```python
from build123d import *

# Parameters (mm, degrees)
SKETCH1_R           = 1
BOSS_EXTRUDE1_DEPTH = 12
SKETCH2_R           = 3.3
CUT_EXTRUDE1_DEPTH  = 4.5
FILLET1_R           = 1
FILLET2_R           = 1
FILLET3_R           = 1
FILLET6_R           = 1


with BuildPart() as part:
    # Sketch1 → Boss-Extrude1 (new body)
    with BuildSketch(Plane.XY):
        with BuildLine():
            Line((0.332668694, 15.169303239), (0.332668694, 22.304947181))
            ThreePointArc((0.332668694, 22.304947181), (-0.167437886, 27.468747249), (4.56623438, 25.3457106))
            Line((4.56623438, 25.3457106), (41.53945423, 8.884172534))
            ThreePointArc((41.53945423, 8.884172534), (44.223987307, 10.459606893), (47.320366603, 10.141571494))
            ThreePointArc((47.320366603, 10.141571494), (47.827175417, 8.821289393), (46.506893317, 8.314480578))
            ThreePointArc((46.506893317, 8.314480578), (42.546047014, 6.794054135), (44.066473458, 2.833207832))
            ThreePointArc((44.066473458, 2.833207832), (44.573282273, 1.512925732), (43.253000172, 1.006116917))
            ThreePointArc((43.253000172, 1.006116917), (40.944771655, 3.094367949), (40.319244301, 6.143536161))
            Line((40.319244301, 6.143536161), (5.332668694, 21.720563222))
            Line((5.332668694, 21.720563222), (5.332668694, 12.544828977))
            Line((5.332668694, 12.544828977), (17.953063304, 7.445858574))
            Line((17.953063304, 7.445858574), (16.829243524, 4.66430701))
            Line((16.829243524, 4.66430701), (3.42965312, 10.078092949))
            ThreePointArc((3.42965312, 10.078092949), (-0.980376986, 10.883023916), (0.332668694, 15.169303239))
        make_face()
        with Locations((1.582668694, 25.03212521)):
            Circle(SKETCH1_R, mode=Mode.SUBTRACT)
        with Locations((1.582668694, 12.44212521)):
            Circle(SKETCH1_R, mode=Mode.SUBTRACT)
    extrude(amount=BOSS_EXTRUDE1_DEPTH)

    # Sketch2 → Cut-Extrude1 (cut)
    with BuildSketch(Plane.XY.offset(12)):
        with Locations((1.582668694, 25.03212521)):
            Circle(SKETCH2_R)
        with Locations((1.582668694, 12.44212521)):
            Circle(SKETCH2_R)
    cut_extrude1 = extrude(amount=-CUT_EXTRUDE1_DEPTH, mode=Mode.SUBTRACT)

    # Mirror1: Cut-Extrude1 across plane
    add(cut_extrude1.mirror(Plane.XY.offset(6)), mode=Mode.SUBTRACT)

    # Fillet1
    fillet1_edges = [part.edges().sort_by_distance(p)[0] for p in [
        (0.332668694, 21.978029599, 9.75),
        (0.332668694, 15.496220821, 9.75),
        (0.332668694, 21.978029599, 2.25),
        (0.332668694, 15.496220821, 2.25),
    ]]
    fillet(fillet1_edges, radius=FILLET1_R)

    # Fillet2
    fillet2_edges = [part.edges().sort_by_distance(p)[0] for p in [
        (17.953063304, 7.445858574, 6),
        (16.829243524, 4.66430701, 6),
    ]]
    fillet(fillet2_edges, radius=FILLET2_R)

    # Fillet3
    fillet3_edges = [part.edges().sort_by_distance(p)[0] for p in [
        (5.332668694, 21.720563222, 6),
        (5.332668694, 12.544828977, 6),
    ]]
    fillet(fillet3_edges, radius=FILLET3_R)

    # Fillet6
    fillet6_edges = [part.edges().sort_by_distance(p)[0] for p in [
        (3.746111613, 9.950235418, 9.75),
        (4.878037932, 25.206886714, 9.75),
        (3.746111613, 9.950235418, 2.25),
        (4.878037932, 25.206886714, 2.25),
    ]]
    fillet(fillet6_edges, radius=FILLET6_R)


solid = part.part
```
Part model, mm, in its own coordinate system. A direction names the side the tool comes from. Coordinates: 2 decimals unless noted, no trailing zeros. Order: outer loops, then holes, each group sorted by start corner. A loop starts at its lowest first (then second) coordinate and runs counter-clockwise, first axis right, second up. Notation, with made-up numbers: (-33, -20.75) - (-5, -20.75) arc R21 cw to (-5, -16.75) - close; hole circle Ø3 at (-15.5, 72). An arc over 180 degrees is marked (long way). Return JSON: item names as keys, results as strings. Group by question number.
Item 1: Cut at B-B (x = 10.5). List the corners of the cut face in (y, z), plus the area to 3 significant figures.
Item 2: Drill centre lines: probe 1 along Y at (x, z) = (5.5, 5.25); probe 2 along X at (y, z) = (17, 7.5); probe 3 along Y at (x, z) = (11.5, 7.5). Where is each one in solid material? Low to high. Write a range as from..to.
Item 3: Cut at C-C (z = 6). List the corners of the cut face in (x, y).
Item 4: Which spindle directions (+Z, -Z, +X, -X, +Y, -Y) get a long thin tool onto all of the face, cutting with end or side? Do faces 1 (the face through (21, 16, 0)), 2 (the face through (23.8, 13.5, 5.9)), 3 (the face through (0.333, 19, 6)). Say none if no direction does.
Item 5: Cut at D-D (y = 23.25). List the corners of the cut face in (x, z), plus the area to 3 significant figures.
Item 6: Pull direction X, two halves, no side cores. Call faces 4 (the face through (2.4, 11.5, 4.5)), 5 (the face through (-0.238, 27.417, 5.979)), 6 (the face through (16.68, 5.05, 6.08)): pulls with the +X half, pulls with the -X half, needs draft (parallel to the pull), parting line crosses it, or undercut.
Item 7: Pin check, flat tips, straight feed: pin 1 (5.5 mm diameter, centred on y = 19.5, z = 4.5, fed in from -X); pin 2 (3 mm diameter, centred on x = 23, z = 10.5, fed in from -Y); pin 3 (3 mm diameter, centred on x = 1.58, y = 25.03, fed in from -Z); pin 4 (12 mm diameter, centred on x = 42.5, y = 19.5, fed in from +Z). Stop position of each tip, or through.
Item 8: Cut at A-A (y = 7.25). List the corners of the cut face in (x, z), plus the area to 3 significant figures.
Check values:
{
 "1": {"outline": "(7.22, 0) - (10.46, 0) - (10.46, 12) - (7.22, 12) - close; (19.42, 0) - (22.7, 0) - (22.7, 12) - (19.42, 12) - close", "area": "78.2 mm2"},
 "2": {"probe 1": "y = 9.24..12.67, 20.73..24.93", "probe 2": "x = 0.33..5.33, 15.94..23.31", "probe 3": "y = 6.82..10.05, 18.97..22.26"},
 "3": {"outline": "(0.33, 15.17) arc R3 ccw (long way) to (3.43, 10.08) - (15.9, 5.04) arc R1 ccw to (17.2, 5.59) - (17.58, 6.52) arc R1 ccw to (17.03, 7.82) - (5.96, 12.29) arc R1 cw to (5.33, 13.22) - (5.33, 20.18) arc R1 cw to (6.74, 21.09) - (40.32, 6.14) arc R5 ccw to (43.25, 1.01) arc R1 ccw to (44.07, 2.83) arc R3 cw to (46.51, 8.31) arc R1 ccw to (47.32, 10.14) arc R5 ccw to (41.54, 8.88) - (4.57, 25.35) arc R3 ccw (long way) to (0.33, 22.3) - close; hole circle Ø2 at (1.58, 12.44); hole circle Ø2 at (1.58, 25.03)"},
 "4": {"face 1": "-Z, +X, -X, +Y, -Y", "face 2": "+Z, -Z", "face 3": "+Z, -Z, -X"},
 "5": {"outline": "(-0.83, 4.5) - (4.36, 4.5) - (4.36, 0) - (9.27, 0) - (9.27, 12) - (4.36, 12) - (4.36, 7.5) - (-0.83, 7.5) - close", "area": "74.5 mm2"},
 "6": {"face 4": "needs draft", "face 5": "parting line crosses it", "face 6": "undercut"},
 "7": {"pin 1": "stops at x = 0.33", "pin 2": "stops at y = 13.19", "pin 3": "stops at z = 4.5", "pin 4": "passes through"},
 "8": {"outline": "(10.43, 0) - (17.59, 0) - (17.59, 12) - (10.43, 12) - close; (37.83, 0) - (42.8, 0) - (42.8, 12) - (37.83, 12) - close", "area": "145 mm2"}
}
